CAD build for the part. Positions are in the model's coordinates, mm. A direction names the side the tool comes from. Coordinates: 2 decimals unless noted, no trailing zeros. Loops run counter-clockwise (first coordinate to the right, second up) from the corner with the lowest first, then second, coordinate; pieces in that order, holes last. Notation, with made-up numbers: (-22, 14) -> (30, 14) arc R3 ccw to (30, 19) -> close; hole circle Ø7 at (81, -21.75). An arc over 180 degrees is marked (long way). Write item = value, one per line. Start each with the question number.
(1) Drill centre lines: line 1 (Y direction, x = 39, z = 12.75); line 2 (X direction, y = 39, z = 13.25); line 3 (X direction, y = -51, z = 17). Where is each one in solid material? Low to high. Write a range as from..to.
(2) Flat gauge pins, fed straight in: P1, Ø6, axis at y = 36, z = 11, coming from the +X side; P2, Ø10, axis at x = -34, y = -51.5, coming from the -Z side; P3, Ø4, axis at x = 7, z = 12.5, coming from the +Y side; P4, Ø0.6, axis at y = -4.5, z = 26.5, coming from the +X side. Where does each tip first touch, or does it go through?
(3) Band-saw the part on A-A (x = 26.5). Write the cut outline in (y, z), and give its area (3 significant figures).
(4) Band-saw the part on C-C (x = 12). Write the cut outline in (y, z).
(5) Tool access for faces 1 (the face through (20.035, -46, 13)), 2 (the face through (18.427, 41, 12)), 3 (the face through (-54.965, -7, 12)): list every direction of +Z, -Z, +X, -X, +Y, -Y with a clear straight run to the whole face (end or side of a thin tool).
(6) Band-saw the part on D-D (z = 7.75). Write the cut outline in (x, y), and give its area (3 significant figures).
(7) Band-saw the part on B-B (y = 46). Write the cut outline in (x, z), and give its area (3 significant figures).
(8) Pull direction Z, two halves, no side cores. Call faces 4 (the face through (32.71, 29.539, 21.747)), 5 (the face through (-6, -66.258, 12)), 6 (the face through (-6, -5, 0)), 7 (the face through (32.71, -35.267, 8.525)): +Z half, -Z half, draft (parallel to the pull), parting line (faces both ways), or undercut.
```python
from build123d import *

# Parameters (mm, degrees)
F0_W     = 100
F0_H     = 120
F1_DEPTH = 25
F2_R     = 11.166084
F3_DEPTH = 25
F4_R     = 10
F5_DEPTH = 25
F7_W     = 95.818966
F7_H     = 109.978452
F8_DEPTH = 2
F6_W     = 42.47845
F6_H     = 5.625
F9_DEPTH = 25


with BuildPart() as f1:
    # F0 (on Top) → F1 (new body)
    with BuildSketch(Plane.XY):
        with Locations((-4.964511, -6.258356)):
            Rectangle(F0_W, F0_H)
    extrude(amount=F1_DEPTH)

    # F2 (on face) → F3 (cut)
    with BuildSketch(Plane.YZ.offset(45.035489)):
        with Locations((-45.5819, 12.801725)):
            Circle(F2_R)
    extrude(amount=-F3_DEPTH, mode=Mode.SUBTRACT)

    # F4 (on face) → F5 (cut)
    with BuildSketch(Plane.YZ.offset(45.035489)):
        with Locations((30.840518, 11.831897)):
            Circle(F4_R)
    extrude(amount=-F5_DEPTH, mode=Mode.SUBTRACT)

    # F7 (on face) → F8 (join)
    with BuildSketch(Plane.XY.offset(25)):
        with Locations((-5.237069, -6.69181)):
            Rectangle(F7_W, F7_H)
    extrude(amount=F8_DEPTH)

    # F6 (on face) → F9 (cut)
    with BuildSketch(Plane(origin=(0, 53.741644, 0), x_dir=(-1, 0, 0), z_dir=(0, 1, 0))):
        with Locations((2.812499, 11.92888)):
            Rectangle(F6_W, F6_H)
    extrude(amount=-F9_DEPTH, mode=Mode.SUBTRACT)


solid = f1.part
```
Findings below:
q1.line_1 = -66.26..-56.75, -34.42..20.88, 40.8..53.74
q1.line_2 = -54.96..-24.05, 18.43..20.04
q1.line_3 = -54.96..20.04
q2.P1 = 20.04
q2.P2 = 0
q2.P3 = 28.74
q2.P4 = 42.67
q3.outline = (-66.26, 0) -> (53.74, 0) -> (53.74, 25) -> (48.3, 25) -> (48.3, 27) -> (-61.68, 27) -> (-61.68, 25) -> (-66.26, 25) -> close; hole circle Ø22.33 at (-45.58, 12.8); hole circle Ø20 at (30.84, 11.83)
q3.area = 2,510 mm²
q4.outline = (-66.26, 0) -> (53.74, 0) -> (53.74, 9.12) -> (28.74, 9.12) -> (28.74, 14.74) -> (53.74, 14.74) -> (53.74, 25) -> (48.3, 25) -> (48.3, 27) -> (-61.68, 27) -> (-61.68, 25) -> (-66.26, 25) -> close
q5.face_1 = +X
q5.face_2 = +Y
q5.face_3 = +Z, -Z, -X, +Y, -Y
q6.outline = (-54.96, -66.26) -> (45.04, -66.26) -> (45.04, -55.54) -> (20.04, -55.54) -> (20.04, -35.62) -> (45.04, -35.62) -> (45.04, 21.71) -> (20.04, 21.71) -> (20.04, 39.97) -> (45.04, 39.97) -> (45.04, 53.74) -> (-54.96, 53.74) -> close
q6.area = 11,000 mm²
q7.outline = (-54.96, 0) -> (45.04, 0) -> (45.04, 25) -> (42.67, 25) -> (42.67, 27) -> (-53.15, 27) -> (-53.15, 25) -> (-54.96, 25) -> close; hole (-24.05, 9.12) -> (18.43, 9.12) -> (18.43, 14.74) -> (-24.05, 14.74) -> close
q7.area = 2,450 mm²
q8.face_4 = undercut
q8.face_5 = draft
q8.face_6 = -Z half
q8.face_7 = undercut
